Can you work these out from the drawing? Everything is in mm from the part's minimum corner. A direction names the side the tool comes from. Give positions to 0.01 mm unless a question says otherwise; leave off trailing zeros. Loops run counter-clockwise (first coordinate to the right, second up) from the corner with the lowest first, then second, coordinate; pieces in that order, holes last.
Q1. I need wall thicknesses on line 1 (X direction, y = 6, z = 4.75) (1 decimal); line 2 (X direction, y = 6, z = 2) (1 decimal); line 3 (X direction, y = 6, z = 4.25) (1 decimal). Which ranges of each line are inside material? Lowest first, please.
Q2. If we section it at B-B (z = 3): Give the number of separate pieces and of enclosed holes in the cut face, plus the area to 3 significant figures.
Q3. If we section it at C-C (x = 17): Please give me the cut outline in (y, z).
Q4. For the marked faces 1 and 2, which set-ups out of +Z, -Z, +X, -X, +Y, -Y let a thin tool reach every point of the face, with its end or its side?
Q5. If we section it at A-A (y = 6): Please give me the cut outline in (x, z) (1 decimal), plus the area to 3 significant figures.
Q6. We'd pull the mould along X, two halves only. Please class the marked faces 3, 4 and 5: +X half, -X half, draft (parallel to the pull), parting line (faces both ways), or undercut.
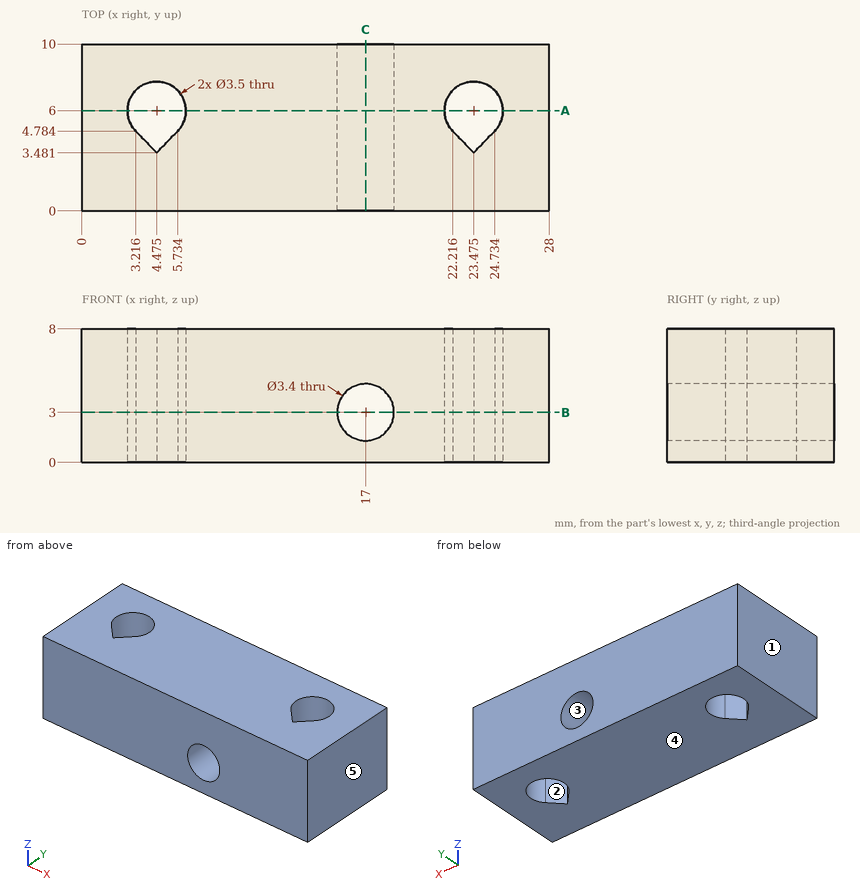
Check sheet entries:
1. line 1: x = 0 to 2.7, 6.2 to 21.7, 25.2 to 28
1. line 2: x = 0 to 2.7, 6.2 to 15.6, 18.4 to 21.7, 25.2 to 28
1. line 3: x = 0 to 2.7, 6.2 to 15.8, 18.2 to 21.7, 25.2 to 28
2. separate pieces: 2
2. enclosed holes: 2
2. area: 225 mm2
3. outline: (0, 0) - (10, 0) - (10, 1.3) - (0, 1.3) - close; (0, 4.7) - (10, 4.7) - (10, 8) - (0, 8) - close
4. face 1: +Z, -Z, -X, +Y, -Y
4. face 2: +Z, -Z
5. outline: (0, 0) - (2.7, 0) - (2.7, 8) - (0, 8) - close; (6.2, 0) - (21.7, 0) - (21.7, 8) - (6.2, 8) - close; (25.2, 0) - (28, 0) - (28, 8) - (25.2, 8) - close; hole circle Ø3.4 at (17, 3)
5. area: 159 mm2
6. face 3: undercut
6. face 4: draft
6. face 5: +X half
